Verification items for the finished model (mm, model axes). Give positions to 0.01 mm unless a question says otherwise; leave off trailing zeros. Order: outer loops, then holes, each group sorted by start corner. A loop starts at its lowest first (then second) coordinate and runs counter-clockwise, first axis right, second up.
(1) Mould release check, pull along Y, two halves, no side actions. Record for faces 1 (the face through (0.882, 22.483, 0.372)), 2 (the face through (0, -2, 0.754)), 3 (the face through (-0.99, 24.98, 0.37)), 4 (the face through (0.871, 29.987, 0.372)): pulls with the +Y half, pulls with the -Y half, needs draft (parallel to the pull), parting line crosses it, or undercut.
(2) Sectioned sample at A-A on y = 5.5. Record the cut outline in (x, z).
(3) Sectioned sample at D-D on z = 0.45. Record the cut outline in (x, y), plus the area to 3 significant figures.
(4) Sectioned sample at C-C on x = -23.5. Record the cut outline in (y, z), plus the area to 3 significant figures.
(5) Gauge pin test, flat end, axial feed: pin 1 (6 mm diameter, centred on x = -6.5, y = 22, fed in from -Z). Record the tip position at first contact, or that the pin passes through.
(6) Sectioned sample at B-B on x = 13. Record the cut outline in (y, z).
(7) Scan lines: L1, parallel to Y at x = -18, z = 0.6; L2, parallel to Y at x = -3.75, z = 0.5; L3, parallel to X at y = 15, z = 0.5. Record each from-to range of solid material in increasing order.
```python
from build123d import *

# Parameters (mm, degrees)
SKETCH1_R           = 0.27178
BOSS_EXTRUDE1_DEPTH = 0.75438


with BuildPart() as part:
    # Sketch1 → Boss-Extrude1 (new body)
    with BuildSketch(Plane.XY):
        with BuildLine():
            Line((-26.292884648, -14.44590658), (-15, -35))
            Line((-15, -35), (-7.5, -35))
            Line((-7.5, -35), (15, -35))
            Line((15, -35), (26.292884648, -14.44590658))
            ThreePointArc((26.292884648, -14.44590658), (0, 30), (-26.292884648, -14.44590658))
        make_face()
        with Locations((-3.750000002, -32.224240034)):
            Circle(SKETCH1_R, mode=Mode.SUBTRACT)
        with Locations((-3.750000002, -26.624240034)):
            Circle(SKETCH1_R, mode=Mode.SUBTRACT)
        Polygon((2.5, -23.848480035), (-2.5, -23.848480035), (-2.5, -22.360679775), (-2.5, -21.213203436), (2.5, -21.213203436), (2.5, -22.360679775), align=None, mode=Mode.SUBTRACT)
        with Locations((-8.733792148, -10)):
            Circle(SKETCH1_R, mode=Mode.SUBTRACT)
        with Locations((-8.733792148, 0)):
            Circle(SKETCH1_R, mode=Mode.SUBTRACT)
        with BuildLine():
            Line((-7.5, -21.213203436), (-7.5, -23.848480035))
            ThreePointArc((-7.5, -23.848480035), (0, 25), (7.5, -23.848480035))
            Line((7.5, -23.848480035), (7.5, -21.213203436))
            ThreePointArc((7.5, -21.213203436), (0, 22.5), (-7.5, -21.213203436))
        make_face(mode=Mode.SUBTRACT)
        with Locations((-8.733792148, 10)):
            Circle(SKETCH1_R, mode=Mode.SUBTRACT)
    extrude(amount=BOSS_EXTRUDE1_DEPTH)


solid = part.part
```
Ans:
1. face 1: undercut
1. face 2: needs draft
1. face 3: undercut
1. face 4: parting line crosses it
2. outline: (-29.49, 0) - (-24.39, 0) - (-24.39, 0.75) - (-29.49, 0.75) - close; (-21.82, 0) - (21.82, 0) - (21.82, 0.75) - (-21.82, 0.75) - close; (24.39, 0) - (29.49, 0) - (29.49, 0.75) - (24.39, 0.75) - close
3. outline: (-26.29, -14.45) - (-15, -35) - (15, -35) - (26.29, -14.45) arc R30 ccw (long way) to start; hole circle Ø0.54 at (-8.73, -10); hole circle Ø0.54 at (-8.73, 0); hole circle Ø0.54 at (-8.73, 10); hole (-7.5, -23.85) - (-7.5, -21.21) arc R22.5 cw (long way) to (7.5, -21.21) - (7.5, -23.85) arc R25 ccw (long way) to start; hole circle Ø0.54 at (-3.75, -32.22); hole circle Ø0.54 at (-3.75, -26.62); hole (-2.5, -23.85) - (2.5, -23.85) - (2.5, -21.21) - (-2.5, -21.21) - close
3. area: 2,750 mm2
4. outline: (-19.53, 0) - (-8.53, 0) - (-8.53, 0.75) - (-19.53, 0.75) - close; (8.53, 0) - (18.65, 0) - (18.65, 0.75) - (8.53, 0.75) - close
4. area: 15.9 mm2
5. pin 1: stops at z = 0
6. outline: (-35, 0) - (-21.35, 0) - (-21.35, 0.75) - (-35, 0.75) - close; (-18.36, 0) - (18.36, 0) - (18.36, 0.75) - (-18.36, 0.75) - close; (21.35, 0) - (27.04, 0) - (27.04, 0.75) - (21.35, 0.75) - close
7. L1: y = -29.54 to -17.35, -13.5 to 13.5, 17.35 to 24
7. L2: y = -35 to -32.5, -31.95 to -26.9, -26.35 to 22.19, 24.72 to 29.76
7. L3: x = -25.98 to -20, -16.77 to 16.77, 20 to 25.98
